Geometry: final body of the model. Coordinates: model frame, mm. A direction names the side the tool comes from. Give positions to 0.01 mm unless a question says otherwise; leave off trailing zeros. Order: outer loops, then holes, each group sorted by start corner. A loop starts at its lowest first (then second) coordinate and runs counter-clockwise, first axis right, second up. Notation, with made-up numbers: (56, 77.25) -> (83, 77.25) arc R22 cw to (83, 101.25) -> close; hole circle Ø2 at (87, 49). An arc over 180 degrees is marked (long way). One line per question, with ' | ' between items.
from build123d import *

# Parameters (mm, degrees)
MAIN_BOARD_OUTLINE_W = 18.5
MAIN_BOARD_OUTLINE_H = 28
SIDE1_DEPTH          = 1
SKETCH2_W            = 2
SKETCH2_H            = 28
WALLS_DEPTH          = 2.3
SKETCH3_R            = 1.5
SCREW_HOLE_DEPTH     = 2.3
SKETCH4_W            = 4.6228
SKETCH4_H            = 2
CUT_EXTRUDE2_DEPTH   = 2.3
SKETCH5_W            = 2
SKETCH5_H            = 4
BOSS_EXTRUDE3_DEPTH  = 2.3


with BuildPart() as part:
    # main board outline → side1 (new body)
    with BuildSketch(Plane(origin=(0, 0, 0), x_dir=(1, 0, 0), z_dir=(0, 1, 0))):
        with Locations((-19.997374583, 0.651042113)):
            Rectangle(MAIN_BOARD_OUTLINE_W, MAIN_BOARD_OUTLINE_H)
    extrude(amount=SIDE1_DEPTH)

    # Sketch2 → walls (add)
    with BuildSketch(Plane(origin=(0, 1, 0), x_dir=(1, 0, 0), z_dir=(0, 1, 0))):
        with Locations((-28.247374583, 0.651042113)):
            Rectangle(SKETCH2_W, SKETCH2_H)
        with Locations((-11.747374583, 0.651042113)):
            Rectangle(SKETCH2_W, SKETCH2_H)
    extrude(amount=WALLS_DEPTH)

    # Sketch3 → screw hole (cut)
    with BuildSketch(Plane(origin=(0, 0, 0), x_dir=(-1, 0, 0), z_dir=(0, -1, 0))):
        with Locations((15.490574583, -10.605757887)):
            Circle(SKETCH3_R)
    extrude(amount=-SCREW_HOLE_DEPTH, mode=Mode.SUBTRACT)

    # Sketch4 → Cut-Extrude2 (cut)
    with BuildSketch(Plane(origin=(0, 0, 0), x_dir=(-1, 0, 0), z_dir=(0, -1, 0))):
        with Locations((21.307174583, -12.348957887)):
            Rectangle(SKETCH4_W, SKETCH4_H)
    extrude(amount=-CUT_EXTRUDE2_DEPTH, mode=Mode.SUBTRACT)

    # Sketch5 → Boss-Extrude3 (add)
    with BuildSketch(Plane(origin=(0, 3.3, 0), x_dir=(1, 0, 0), z_dir=(0, 1, 0))):
        with Locations((-28.247374583, 8.651042113)):
            Rectangle(SKETCH5_W, SKETCH5_H)
        with Locations((-28.247374583, -4.348957887)):
            Rectangle(SKETCH5_W, SKETCH5_H)
        with Locations((-11.747374583, 8.651042113)):
            Rectangle(SKETCH5_W, SKETCH5_H)
        with Locations((-11.747374583, -4.348957887)):
            Rectangle(SKETCH5_W, SKETCH5_H)
    extrude(amount=BOSS_EXTRUDE3_DEPTH)


solid = part.part
1) Contact query for flat-ended pins moving along their axis: pin 1 Ø1 at (x, y) = (-28, 5) entering from +Z; pin 2 Ø3.5 at (x, z) = (-15.49, 10.61) entering from +Y; pin 3 Ø3 at (x, y) = (-26, 2) entering from -Z; pin 4 Ø0.8 at (x, y) = (-21.5, 0.5) entering from +Z. Output: stop coordinate, or through.
Check result:
pin 1: stops at z = 6.35 | pin 2: stops at y = 1 | pin 3: stops at z = -14.65 | pin 4: stops at z = 11.35
2) Section A-A on y = 3. Return loops of the section in (x, z).
Check result:
outline: (-29.25, -14.65) -> (-27.25, -14.65) -> (-27.25, 13.35) -> (-29.25, 13.35) -> close; (-12.75, -14.65) -> (-10.75, -14.65) -> (-10.75, 13.35) -> (-12.75, 13.35) -> close
3) Pull-direction query (Z, two-part tool) for faces 4 (the flat face through (-12, 4, -6.651)), 5 (the flat face through (-12, 4, -10.651)), 6 (the flat face through (-28, 4, 6.349)); classes: +Z half, -Z half, draft (parallel to the pull), parting line (faces both ways), or undercut.
Check result:
face 4: undercut | face 5: -Z half | face 6: +Z half
4) Section C-C on x = -16.5. Return loops of the section in (y, z), plus the area to 3 significant figures.
Check result:
outline: (0, -14.65) -> (1, -14.65) -> (1, 9.5) -> (0, 9.5) -> close; (0, 11.72) -> (1, 11.72) -> (1, 13.35) -> (0, 13.35) -> close | area: 25.8 mm^2
5) Section B-B on z = -5. Return loops of the section in (x, y), plus the area to 3 significant figures.
Check result:
outline: (-29.25, 0) -> (-10.75, 0) -> (-10.75, 3.3) -> (-12.75, 3.3) -> (-12.75, 1) -> (-27.25, 1) -> (-27.25, 3.3) -> (-29.25, 3.3) -> close | area: 27.7 mm^2
6) Section D-D on y = 0.7. Return loops of the section in (x, z).
Check result:
outline: (-29.25, -14.65) -> (-10.75, -14.65) -> (-10.75, 13.35) -> (-19, 13.35) -> (-19, 11.35) -> (-23.62, 11.35) -> (-23.62, 13.35) -> (-29.25, 13.35) -> close; hole circle Ø3 at (-15.49, 10.61)
7) Set-up query: faces 1 (the flat face through (-12, 3.3, 10)), 2 (the flat face through (-18.996, 0.5, 12.4)), 3 (the flat face through (-28, 4, 2.349)). Return all of +Z, -Z, +X, -X, +Y, -Y with unobstructed straight access to the full face (end or side cutting, diameter ignored); none if empty.
Check result:
face 1: +Z, +X, -X, +Y | face 2: +Z, +Y, -Y | face 3: +X, -X, +Y
8) Material intervals for probe 1 along X at (y, z) = (3.15, 6.5); probe 2 along Z at (x, y) = (-12.5, 5); probe 3 along Y at (x, z) = (-28, 1.5), sorted ascending. Write a range as from..to.
Check result:
probe 1: x = -29.25..-27.25, -12.75..-10.75 | probe 2: z = -10.65..-6.65, 2.35..6.35 | probe 3: y = 0..3.3
